The model under review builds one solid part; all positions refer to its coordinate system, in mm. Coordinates: 2 decimals unless noted, no trailing zeros. Write each loop counter-clockwise with the first axis right and the second up, starting at its lowest first coordinate (ties: lowest second). Pieces come first, ordered by that corner, then holes.
1) Add section D-D, the plane x = -7.75. State the section outline as (y, z) points.
2) Add section A-A, the plane x = 0. State the section outline as (y, z) points (3 decimals).
3) Add section B-B, the plane y = 0.5. State the section outline as (x, z) points (3 decimals), then the cut area to 3 significant figures.
4) Add section C-C, the plane z = -24.5. State the section outline as (x, y) points (3 decimals).
5) For line 1 (Z direction, x = 0, y = 5.5) (3 decimals); line 2 (Z direction, x = -1.5, y = 4.5); line 3 (X direction, y = 5.5, z = -26), list the stretches that pass through material, from the lowest coordinate up.
6) Mouldability with a two-part tool opening along X and no side actions: class faces 1 (the flat face through (-9.525, 3, -13)), 2 (the cylindrical face through (0.28, 3.48, -2.14)), 3 (the cylindrical face through (-0.209, 3.481, -34.923)) as released by +X, released by -X, zero draft, split by the parting line, or undercut.
7) For P1, Ø3, axis at x = -6, y = 3.5, coming from the +Z side (3 decimals), flat-tipped, find the tip position at first contact; note if it passes through.
Autodesk Inventor part; units mm, degrees
ref_plane "YZ Plane" through (0, 0, 0) normal (1, 0, 0) x (0, 1, 0)
ref_plane "XZ Plane" through (0, 0, 0) normal (0, 1, 0) x (-1, 0, 0)
ref_plane "XY Plane" through (0, 0, 0) normal (0, 0, 1) x (1, 0, 0)
sketch "Sketch1" plane through (0, 0, 0) normal (0, 1, 0) x (-1, 0, 0)
  circle A0 centre (0, 0) radius 2.159
  circle A1 centre (0, -25.4) radius 2.159
  line L0 (0, 0) -> (0, -25.4) construction
  line L1 (-9.525, 0) -> (-9.525, -25.4)
  line L2 (9.525, -25.4) -> (9.525, 0)
  arc A2 (9.525, 0) -> (-9.525, 0) centre (0, 0) ccw
  arc A3 (-9.525, -25.4) -> (9.525, -25.4) centre (0, -25.4) ccw
  point P0 (0, -12.7)
  dimension "d0" = 4.318
  dimension "d2" = 25.4
  dimension "d3" = 19.05
extrude "Extrusion1" add sketch "Sketch1" along normal blind 7.061
properties part number "Large Motor Spacer" material "PET Plastic"
Geometry results:
1. outline: (0, -30.94) - (7.06, -30.94) - (7.06, 5.54) - (0, 5.54) - close
2. outline: (0, -34.925) - (7.061, -34.925) - (7.061, -27.559) - (0, -27.559) - close; (0, -23.241) - (7.061, -23.241) - (7.061, -2.159) - (0, -2.159) - close; (0, 2.159) - (7.061, 2.159) - (7.061, 9.525) - (0, 9.525) - close
3. outline: (-9.525, -25.4) arc R9.525 ccw to (9.525, -25.4) - (9.525, 0) arc R9.525 ccw to (-9.525, 0) - close; hole circle Ø4.318 at (0, -25.4); hole circle Ø4.318 at (0, 0)
3. area: 740 mm2
4. outline: (-9.525, 0) - (-1.962, 0) - (-1.962, 7.061) - (-9.525, 7.061) - close; (1.962, 0) - (9.525, 0) - (9.525, 7.061) - (1.962, 7.061) - close
5. line 1: z = -34.925 to -27.559, -23.241 to -2.159, 2.159 to 9.525
5. line 2: z = -34.81 to -26.95, -23.85 to -1.55, 1.55 to 9.41
5. line 3: x = -9.51 to -2.07, 2.07 to 9.51
6. face 1: released by -X
6. face 2: undercut
6. face 3: split by the parting line
7. P1: stops at z = 8.395
